Design review of the part built by this model. Coordinates are the model's own, in mm. A direction names the side the tool comes from. Give positions to 0.01 mm unless a question says otherwise; leave off trailing zeros. Write each loop counter-clockwise with the first axis right and the second up, starting at its lowest first coordinate (ties: lowest second). Pieces come first, ordered by that corner, then holes. Notation, with made-up numbers: (-11.75, 30) -> (33.25, 30) arc R8 ccw to (33.25, 41) -> close; hole circle Ø1 at (-6.5, 59.25). An arc over 180 degrees is marked (long way). Return JSON: item names as keys, results as strings. Group by question number.
from build123d import *

# Parameters (mm, degrees)
SKETCH2_R           = 10
BOSS_EXTRUDE1_DEPTH = 50
CUT_EXTRUDE3_DEPTH  = 88.648445508
SKETCH5_R           = 5
BOSS_EXTRUDE2_DEPTH = 6


with BuildPart() as part:
    # Sketch2 → Boss-Extrude1 (new, symmetric)
    with BuildSketch(Plane(origin=(0, 0, 0), x_dir=(0, 0, -1), z_dir=(1, 0, 0))):
        Circle(SKETCH2_R)
    extrude(amount=BOSS_EXTRUDE1_DEPTH, both=True)

    # Sketch4 → Cut-Extrude3 (cut, through all)
    with BuildSketch(Plane(origin=(-36.5, 0, 0), x_dir=(0, 0, -1), z_dir=(1, 0, 0))):
        with BuildLine():
            Line((7.353740545, -3.15), (9.49091671, -3.15))
            ThreePointArc((9.49091671, -3.15), (10, 0), (9.49091671, 3.15))
            Line((9.49091671, 3.15), (7.353740545, 3.15))
            ThreePointArc((7.353740545, 3.15), (8, 0), (7.353740545, -3.15))
        make_face()
        with BuildLine():
            Line((-7.473438377, 6.644374976), (-6.404850294, 4.793526125))
            ThreePointArc((-6.404850294, 4.793526125), (-4, 6.92820323), (-0.94889025, 7.943526125))
            Line((-0.94889025, 7.943526125), (-2.017478333, 9.794374976))
            ThreePointArc((-2.017478333, 9.794374976), (-5, 8.660254038), (-7.473438377, 6.644374976))
        make_face()
        with BuildLine():
            Line((-9.49091671, -3.15), (-7.353740545, -3.15))
            ThreePointArc((-7.353740545, -3.15), (-8, 0), (-7.353740545, 3.15))
            Line((-7.353740545, 3.15), (-9.49091671, 3.15))
            ThreePointArc((-9.49091671, 3.15), (-10, 0), (-9.49091671, -3.15))
        make_face()
        with BuildLine():
            Line((-2.017478333, -9.794374976), (-0.94889025, -7.943526125))
            ThreePointArc((-0.94889025, -7.943526125), (-4, -6.92820323), (-6.404850294, -4.793526125))
            Line((-6.404850294, -4.793526125), (-7.473438377, -6.644374976))
            ThreePointArc((-7.473438377, -6.644374976), (-5, -8.660254038), (-2.017478333, -9.794374976))
        make_face()
        with BuildLine():
            Line((0.94889025, -7.943526125), (2.017478333, -9.794374976))
            ThreePointArc((2.017478333, -9.794374976), (5, -8.660254038), (7.473438377, -6.644374976))
            Line((7.473438377, -6.644374976), (6.404850294, -4.793526125))
            ThreePointArc((6.404850294, -4.793526125), (4, -6.92820323), (0.94889025, -7.943526125))
        make_face()
        with BuildLine():
            Line((6.404850294, 4.793526125), (7.473438377, 6.644374976))
            ThreePointArc((7.473438377, 6.644374976), (5, 8.660254038), (2.017478333, 9.794374976))
            Line((2.017478333, 9.794374976), (0.94889025, 7.943526125))
            ThreePointArc((0.94889025, 7.943526125), (4, 6.92820323), (6.404850294, 4.793526125))
        make_face()
    cut_extrude3 = extrude(amount=-CUT_EXTRUDE3_DEPTH, mode=Mode.SUBTRACT)

    # Sketch5 → Boss-Extrude2 (add)
    with BuildSketch(Plane.ZY.offset(50)):
        Circle(SKETCH5_R)
    boss_extrude2 = extrude(amount=BOSS_EXTRUDE2_DEPTH)

    # Mirror3: Cut-Extrude3, Boss-Extrude2 across plane
    add(cut_extrude3.mirror(Plane(origin=(0, 0, 0), x_dir=(0, 0, 1), z_dir=(1, 0, 0))), mode=Mode.SUBTRACT)
    add(boss_extrude2.mirror(Plane(origin=(0, 0, 0), x_dir=(0, 0, 1), z_dir=(1, 0, 0))))


solid = part.part
Q1. Mouldability with a two-part tool opening along Z and no side actions: class faces 3 (the face through (-43.156, 5.706, -6.932)), 4 (the face through (-36.5, 0, -9)) as +Z half, -Z half, draft (parallel to the pull), parting line (faces both ways), or undercut.
Q2. For L1, parallel to X at y = -8, z = -2.25; L2, parallel to X at y = 3.5, z = -7.5; L3, parallel to Y at x = -8, z = 0.5, list the stretches that pass through material, from the lowest coordinate up. Write a range as from..to.
Q3. Take a section at B-B, the plane z = 0. Give the boundary of the cut face in (x, y).
Q4. Take a section at C-C, the plane y = 0. Give the boundary of the cut face in (x, z).
Q5. Tool access review of faces 1 (the face through (36.5, -8, -4)), 2 (the face through (-36.5, -8, -4)): name each direction out of +Z, -Z, +X, -X, +Y, -Y from which nothing blocks a thin tool from reaching the whole face with its end or side.
Q6. Insertion check: pin 1 (4 mm diameter, centred on y = 8, z = -5, fed in from -X); pin 2 (2.5 mm diameter, centred on y = -7.5, z = 4, fed in from +X); pin 3 (0.6 mm diameter, centred on x = 42, z = -8.5, fed in from +Y). Each pin has a flat end and moves straight along its axis. Give the tip position at first contact, or say it passes through.
Q7. Take a section at A-A, the plane x = -39. Give the boundary of the cut face in (y, z).
Final values:
{
 "1": {"face 3": "undercut", "face 4": "draft"},
 "2": {"L1": "x = -36.5..36.5", "L2": "x = -50..50", "L3": "y = -9.99..9.99"},
 "3": {"outline": "(-56, -5) -> (-50, -5) -> (-50, -10) -> (50, -10) -> (50, -5) -> (56, -5) -> (56, 5) -> (50, 5) -> (50, 10) -> (-50, 10) -> (-50, 5) -> (-56, 5) -> close"},
 "4": {"outline": "(-56, -5) -> (-50, -5) -> (-50, -8) -> (-36.5, -8) -> (-36.5, -10) -> (36.5, -10) -> (36.5, -8) -> (50, -8) -> (50, -5) -> (56, -5) -> (56, 5) -> (50, 5) -> (50, 8) -> (36.5, 8) -> (36.5, 10) -> (-36.5, 10) -> (-36.5, 8) -> (-50, 8) -> (-50, 5) -> (-56, 5) -> close"},
 "5": {"face 1": "+X", "face 2": "-X"},
 "6": {"pin 1": "stops at x = -50", "pin 2": "stops at x = 50", "pin 3": "stops at y = 5.72"},
 "7": {"outline": "(-9.79, -2.02) -> (-7.94, -0.95) arc R8 ccw to (-4.79, -6.4) -> (-6.64, -7.47) arc R10 ccw to (-3.15, -9.49) -> (-3.15, -7.35) arc R8 ccw to (3.15, -7.35) -> (3.15, -9.49) arc R10 ccw to (6.64, -7.47) -> (4.79, -6.4) arc R8 ccw to (7.94, -0.95) -> (9.79, -2.02) arc R10 ccw to (9.79, 2.02) -> (7.94, 0.95) arc R8 ccw to (4.79, 6.4) -> (6.64, 7.47) arc R10 ccw to (3.15, 9.49) -> (3.15, 7.35) arc R8 ccw to (-3.15, 7.35) -> (-3.15, 9.49) arc R10 ccw to (-6.64, 7.47) -> (-4.79, 6.4) arc R8 ccw to (-7.94, 0.95) -> (-9.79, 2.02) arc R10 ccw to start"}
}
